```python
from build123d import *

# Parameters (mm, degrees)
SKETCH_1_R          = 3
EXTRUDE_1_DEPTH     = 3
SKETCH_2_R          = 1.5
CUT_EXTRUDE_1_DEPTH = 0.6
CUT_EXTRUDE_2_DEPTH = 1.1


with BuildPart() as part:
    # 草图1 → 凸台-拉伸1 (new body)
    with BuildSketch(Plane.XY):
        Circle(SKETCH_1_R)
    extrude(amount=EXTRUDE_1_DEPTH)

    # 草图2 → 切除-拉伸1 (cut)
    with BuildSketch(Plane.XY.offset(3)):
        Circle(SKETCH_2_R)
    extrude(amount=-CUT_EXTRUDE_1_DEPTH, mode=Mode.SUBTRACT)

    # 草图3 → 切除-拉伸2 (cut)
    with BuildSketch(Plane.XY.offset(2.4)):
        with BuildLine():
            Line((-1.075103849, 2.800741279), (-1.343879811, 3.500926599))
            ThreePointArc((-1.343879811, 3.500926599), (2.651650429, 2.651650429), (3.500926599, -1.343879811))
            Line((3.500926599, -1.343879811), (2.800741279, -1.075103849))
            ThreePointArc((2.800741279, -1.075103849), (2.527515353, -0.46142837), (1.913839874, -0.734654297))
            ThreePointArc((1.913839874, -0.734654297), (-1.449568901, -1.449568901), (-0.734654297, 1.913839874))
            ThreePointArc((-0.734654297, 1.913839874), (-0.46142837, 2.527515353), (-1.075103849, 2.800741279))
        make_face()
    extrude(amount=-CUT_EXTRUDE_2_DEPTH, mode=Mode.SUBTRACT)


solid = part.part
```
Geometry: final body of the model. Coordinates: model frame, mm. A direction names the side the tool comes from. Round coordinates to 2 decimals unless told otherwise and drop trailing zeros. Write each loop counter-clockwise with the first axis right and the second up, starting at its lowest first coordinate (ties: lowest second). Pieces come first, ordered by that corner, then holes. Notation, with made-up numbers: (-18.75, 73) -> (7.25, 73) arc R31 ccw to (7.25, 102) -> close; hole circle Ø3 at (26, 24.5). An arc over 180 degrees is marked (long way). Return JSON: item names as keys, results as strings.
Q1. Section A-A on x = 0. Return the cut outline in (y, z).
From the geometry:
{"outline": "(-3, 0) -> (3, 0) -> (3, 1.3) -> (-2.05, 1.3) -> (-2.05, 2.4) -> (-1.5, 2.4) -> (-1.5, 3) -> (-3, 3) -> close; (1.5, 2.4) -> (3, 2.4) -> (3, 3) -> (1.5, 3) -> close"}
Q2. Mould query, pull axis X, two halves, no side actions, for faces 3 (the cylindrical face through (-1.5, 0.07, 2.7)), 4 (the cylindrical face through (-0.65, -2.93, 1.48)), 5 (the flat face through (1.3, -1.3, 3)). Classes: +X half, -X half, draft (parallel to the pull), parting line (faces both ways), or undercut.
From the geometry:
{"face 3": "undercut", "face 4": "parting line", "face 5": "draft"}
Q3. First-contact query: pin 1 Ø1 at (x, y) = (-0.5, -0.5) entering from +Z; pin 2 Ø1 at (x, z) = (2, 0.5) entering from +Y. Flat tips, straight axial feed; report the tip coordinate or a pass-through.
From the geometry:
{"pin 1": "z = 1.3", "pin 2": "y = 2.6"}
Q4. Set-up query: faces 1 (the flat face through (1, 1, 1.3)), 2 (the flat face through (0, 0, 0)). Return all of +Z, -Z, +X, -X, +Y, -Y with unobstructed straight access to the full face (end or side cutting, diameter ignored); none if empty.
From the geometry:
{"face 1": "none", "face 2": "-Z, +X, -X, +Y, -Y"}
Q5. Section D-D on z = 0.3. Return the cut outline in (x, y), and give its area (3 significant figures).
From the geometry:
{"outline": "circle Ø6 at (0, 0)", "area": "28.3 mm2"}
Q6. Ray query, line 1 (Z direction, x = 1.2, y = 1.95); line 2 (Y direction, x = 0, z = 2.75); line 3 (Z direction, x = -0.55, y = -0.85). Return the intervals inside material, ascending.
From the geometry:
{"line 1": "0 to 1.3, 2.4 to 3", "line 2": "-3 to -1.5, 1.5 to 3", "line 3": "0 to 1.3"}
